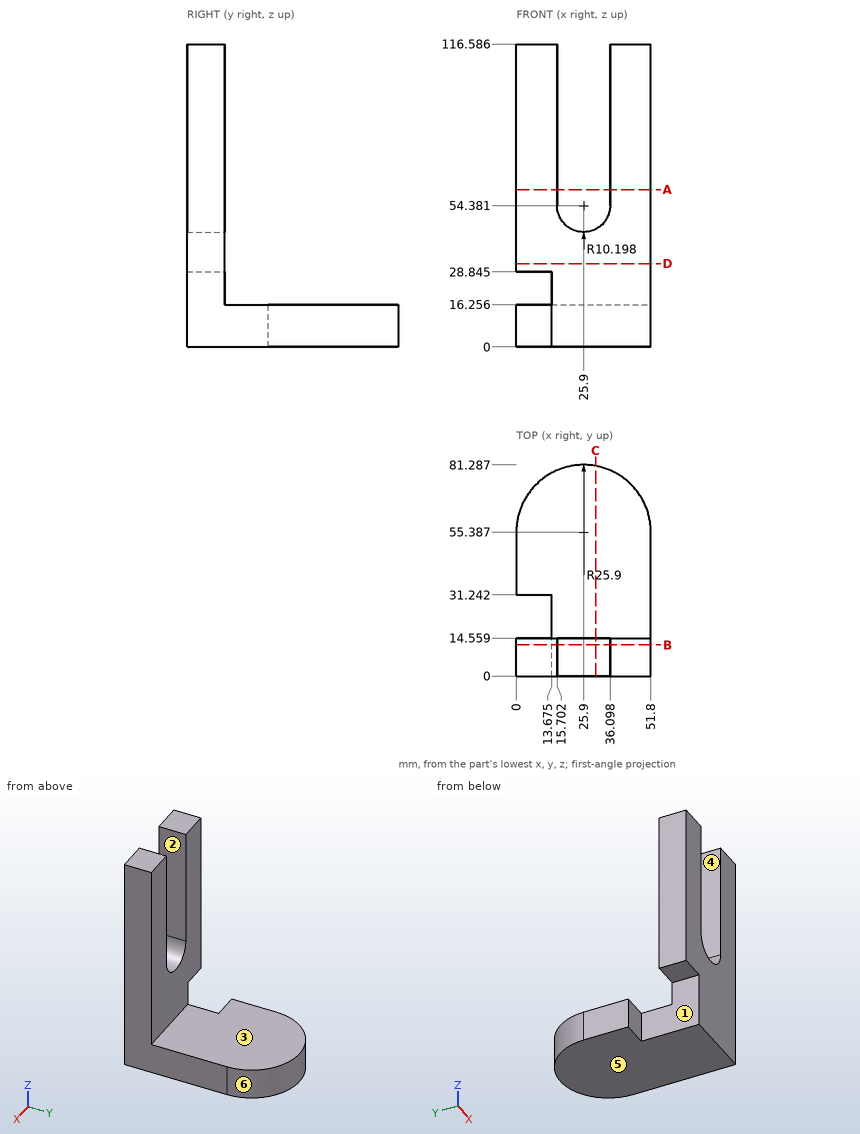
The figure shows three views and two pictorial views of one solid part (mm, origin at its lowest corner). Answer the questions. A direction names the side the tool comes from. Give positions to 0.01 mm unless a question says otherwise; leave off trailing zeros. Order: outer loops, then holes, each group sorted by start corner. A loop starts at its lowest first (then second) coordinate and runs counter-clockwise, first axis right, second up. Notation, with made-up numbers: (51, 17.25) -> (108, 17.25) arc R35 ccw to (108, 56.25) -> close; hole circle Ø3 at (9.5, -34). An arc over 180 degrees is marked (long way). Answer as a JSON object with one key per item and string values. Group by question number.
Item 1: The part is cut by section D-D on z = 32. Write down the section's boundary in (x, y), and give its area (3 significant figures).
Item 2: Determine the mould class of the marked faces 4, 5 and 6 for opening direction X: pulls with the +X half, pulls with the -X half, needs draft (parallel to the pull), parting line crosses it, or undercut.
Item 3: The part is cut by section B-B on y = 12. Write down the section's boundary in (x, z) (1 decimal), and give its area (3 significant figures).
Item 4: A tool of negligible diameter and unlimited length cuts with its end or side. For the marked faces 1, 2 and 3, from which of +Z, -Z, +X, -X, +Y, -Y can it reach the whole face along a straight path? Write none if from no direction.
Item 5: Flat-ended cylindrical pins translate along their axes: pin 1 (8.5 mm diameter, centred on y = 13, z = 17, fed in from -X) (1 decimal); pin 2 (5 mm diameter, centred on x = 40.5, z = 66, fed in from -Y); pin 3 (4 mm diameter, centred on x = 37.5, y = 66, fed in from +Z); pin 4 (15 mm diameter, centred on x = 4.5, y = 8.5, fed in from -Z) (3 decimals). Find the tip coordinate at first contact, or state that the pin passes through.
Item 6: Consider L1, parallel to Y at x = 44, z = 77; L2, parallel to X at y = 5.5, z = 45 (1 decimal); L3, parallel to Z at x = 28, y = 41. Determine where each line is inside the solid, lowest interval first. Write a range as from..to.
Item 7: The part is cut by section C-C on x = 30.5. Write down the section's boundary in (y, z) (1 decimal), and give its area (3 significant figures).
Item 8: The part is cut by section A-A on z = 60.5. Write down the section's boundary in (x, y).
Result set:
{
 "1": {"outline": "(0, 0) -> (51.8, 0) -> (51.8, 14.56) -> (0, 14.56) -> close", "area": "754 mm²"},
 "2": {"face 4": "undercut", "face 5": "needs draft", "face 6": "parting line crosses it"},
 "3": {"outline": "(0, 28.8) -> (13.7, 28.8) -> (13.7, 0) -> (51.8, 0) -> (51.8, 116.6) -> (36.1, 116.6) -> (36.1, 54.4) arc R10.2 cw to (15.7, 54.4) -> (15.7, 116.6) -> (0, 116.6) -> close", "area": "4,210 mm²"},
 "4": {"face 1": "-Z, -X, -Y", "face 2": "+Z, +Y, -Y", "face 3": "+Z, +X, -X, +Y"},
 "5": {"pin 1": "x = 13.7", "pin 2": "y = 0", "pin 3": "z = 16.26", "pin 4": "z = 28.845"},
 "6": {"L1": "0..14.56", "L2": "0..21.9, 29.9..51.8", "L3": "0..16.26"},
 "7": {"outline": "(0, 0) -> (80.9, 0) -> (80.9, 16.3) -> (14.6, 16.3) -> (14.6, 45.3) -> (0, 45.3) -> close", "area": "1,740 mm²"},
 "8": {"outline": "(0, 0) -> (15.7, 0) -> (15.7, 14.56) -> (0, 14.56) -> close; (36.1, 0) -> (51.8, 0) -> (51.8, 14.56) -> (36.1, 14.56) -> close"}
}
